```python
from build123d import *

# Parameters (mm, degrees)
F1_DEPTH = 150
F2_R     = 120
F3_DEPTH = 270
F4_W     = 717.304408
F4_H     = 111.2508
F4_W_2   = 697.326451
F4_H_2   = 148.352754
F5_DEPTH = 160
F6_W     = 120
F6_H     = 100
F7_DEPTH = 100
F9_DEPTH = 450.001


with BuildPart() as f1:
    # F0 (on Front) → F1 (new body, symmetric)
    with BuildSketch(Plane.XZ):
        Polygon((-225, -75), (225, -75), (225, -35), (120, 75), (-120, 75), (-225, -35), align=None)
    extrude(amount=F1_DEPTH, both=True)

    # F2 (on face) → F3 (join)
    with BuildSketch(Plane.XY.offset(75)):
        Circle(F2_R)
    extrude(amount=F3_DEPTH)

    # F4 (on face) → F5 (cut)
    with BuildSketch(Plane.XY.offset(345)):
        with Locations((0, 105.6254)):
            Rectangle(F4_W, F4_H)
        with Locations((9.988979, -124.176377)):
            Rectangle(F4_W_2, F4_H_2)
    extrude(amount=-F5_DEPTH, mode=Mode.SUBTRACT)

    # F6 (on face) → F7 (cut)
    with BuildSketch(Plane.XY.offset(345)):
        Rectangle(F6_W, F6_H)
    extrude(amount=-F7_DEPTH, mode=Mode.SUBTRACT)

    # F8 (on face) → F9 (cut, through all)
    with BuildSketch(Plane.YZ.offset(225)):
        Polygon((-30, -35), (-30, -75), (30, -75), (30, -35), (75, 0), (75, 30), (-75, 30), (-75, 0), align=None)
    extrude(amount=-F9_DEPTH, mode=Mode.SUBTRACT)


solid = f1.part
```
The listing builds one solid part. Answer for the finished solid, in the listing's coordinates (mm). A direction names the side the tool comes from. Coordinates: 2 decimals unless noted, no trailing zeros. Write each loop counter-clockwise with the first axis right and the second up, starting at its lowest first coordinate (ties: lowest second). Pieces come first, ordered by that corner, then holes. Notation, with made-up numbers: (22, 25) - (48, 25) arc R33 cw to (48, 60) - close; hole circle Ø9 at (67.25, 9). An arc over 180 degrees is marked (long way). Return JSON: item names as keys, results as strings. Group by question number.
Q1. Find the intervals of material crossed by line 1 along Z through (x, y) = (-87, -89.5); line 2 along Z through (x, y) = (-66, 2.5); line 3 along X through (y, z) = (22, 266), in increasing order. Write a range as [from, to].
Q2. Flat-ended cylindrical pins translate along their axes: pin 1 Ø12 at (x, z) = (-95, 143.5) entering from -Y; pin 2 Ø3 at (y, z) = (-112.5, 74.5) entering from +X; pin 3 Ø2 at (y, z) = (23.5, 149.5) entering from -X. Find the tip coordinate at first contact, or state that the pin passes through.
Q3. The part is cut by section D-D on z = 233. Write down the section's boundary in (x, y), and give its area (3 significant figures).
Q4. The part is cut by section C-C on x = 0. Write down the section's boundary in (y, z).
Q5. The part is cut by section B-B on z = 306. Write down the section's boundary in (x, y), and give its area (3 significant figures).
Q6. The part is cut by section A-A on y = -62. Write down the section's boundary in (x, z), and give its area (3 significant figures).
Q7. Which of the six approach directions +Z, -Z, +X, -X, +Y, -Y give full straight-line access (tool end or side, diameter ignored) to faces 1 (the flat face through (-2, -77, 185)), 2 (the flat face through (3, -30, -55)), 3 (the flat face through (1, 125, 75)), 4 (the cylindrical face through (110.85, -45.96, 178.11)), 5 (the flat face through (3.15, -52.815, -17.255))?
Q8. For a pull along X with two mould halves and no side action, classify faces 6 (the flat face through (-1, 1, 245)), 7 (the flat face through (162, -2, 31)), 8 (the flat face through (-3, -150, -16)) as +X half, -X half, draft (parallel to the pull), parting line (faces both ways), or undercut.
Evaluation:
{
 "1": {"line 1": "z = [-75, 75]", "line 2": "z = [30, 345]", "line 3": "x = [-117.97, -60], [60, 117.97]"},
 "2": {"pin 1": "stops at y = -80.49", "pin 2": "stops at x = 121.91", "pin 3": "stops at x = -117.87"},
 "3": {"outline": "(-109.09, -50) - (109.09, -50) arc R120 ccw to (109.09, 50) - (-109.09, 50) arc R120 ccw to start", "area": "23,300 mm2"},
 "4": {"outline": "(-150, -75) - (-30, -75) - (-30, -35) - (-75, 0) - (-75, 30) - (75, 30) - (75, 0) - (30, -35) - (30, -75) - (150, -75) - (150, 75) - (120, 75) - (120, 185) - (50, 185) - (50, 245) - (-50, 245) - (-50, 185) - (-120, 185) - (-120, 75) - (-150, 75) - close"},
 "5": {"outline": "(-109.09, -50) - (-60, -50) - (-60, 50) - (-109.09, 50) arc R120 ccw to start; (60, -50) - (109.09, -50) arc R120 ccw to (109.09, 50) - (60, 50) - close", "area": "11,300 mm2"},
 "6": {"outline": "(-225, -75) - (225, -75) - (225, -35) - (201.24, -10.11) - (-201.24, -10.11) - (-225, -35) - close; (-162.95, 30) - (162.95, 30) - (120, 75) - (102.74, 75) - (102.74, 185) - (-102.74, 185) - (-102.74, 75) - (-120, 75) - close", "area": "63,900 mm2"},
 "7": {"face 1": "+Z, +X, -X, -Y", "face 2": "-Z, +X, -X", "face 3": "+Z, +Y", "face 4": "+Z", "face 5": "+X, -X"},
 "8": {"face 6": "undercut", "face 7": "+X half", "face 8": "draft"}
}
